Part model, mm, in its own coordinate system. Give positions to 0.01 mm unless a question says otherwise; leave off trailing zeros. Write each loop counter-clockwise with the first axis right and the second up, starting at its lowest first coordinate (ties: lowest second). Pieces come first, ordered by that corner, then holes. Notation, with made-up numbers: M 81.25,-31.5 L 96.25,-31.5 A30 cw 96.25,-3.5 Z; hole C 40,26 d10. An arc over 180 degrees is marked long. Use a Markdown table: item, result. Add a question column.
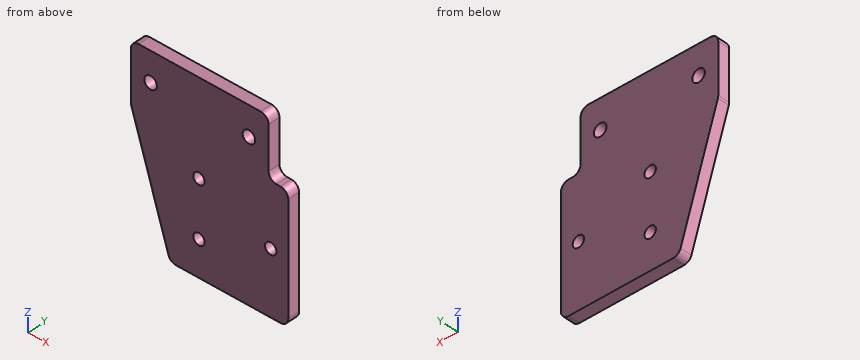
from build123d import *

# Parameters (mm, degrees)
SKETCH_1_R      = 1.6
SKETCH_1_R_2    = 1.45
EXTRUDE_1_DEPTH = 3
FILLET_2_R      = 2


with BuildPart() as part:
    # 草图1 → 凸台-拉伸1 (new body)
    with BuildSketch(Plane(origin=(0, 0, 0), x_dir=(1, 0, 0), z_dir=(0, 1, 0))):
        Polygon((0, 0), (0, 15), (10, 47), (25, 47), (40, 47), (40, 15), (35, 15), (35, 0), align=None)
        with Locations(Location((30, 7.5, 0), (0, 0, 270))):
            Circle(SKETCH_1_R, mode=Mode.SUBTRACT)
        with Locations(Location((5, 7.5, 0), (0, 0, 90))):
            Circle(SKETCH_1_R, mode=Mode.SUBTRACT)
        with Locations(Location((35.551575044, 30.824296308, 0), (0, 0, 270))):
            Circle(SKETCH_1_R_2, mode=Mode.SUBTRACT)
        with Locations(Location((17.301575044, 37.924296308, 0), (0, 0, 270))):
            Circle(SKETCH_1_R_2, mode=Mode.SUBTRACT)
        with Locations(Location((17.301575044, 23.724296308, 0), (0, 0, 270))):
            Circle(SKETCH_1_R_2, mode=Mode.SUBTRACT)
    extrude(amount=EXTRUDE_1_DEPTH)

    # 圆角2
    fillet_2_edges = [part.edges().sort_by_distance(p)[0] for p in [
        (35, 1.5, -15),
        (35, 1.5, 0),
        (0, 1.5, 0),
        (0, 1.5, -15),
        (10, 1.5, -47),
        (40, 1.5, -47),
        (40, 1.5, -15),
    ]]
    fillet(fillet_2_edges, radius=FILLET_2_R)


solid = part.part
1. Flat gauge pins, fed straight in: pin 1 (1 mm diameter, centred on y = 2.5, z = -23.5, fed in from -X); pin 2 (2.5 mm diameter, centred on x = 17.3, z = -37.92, fed in from -Y); pin 3 (1.1 mm diameter, centred on x = 37.5, y = 2, fed in from +Z); pin 4 (1.5 mm diameter, centred on y = 1.5, z = -23, fed in from -X). Where does each tip first touch, or does it go through?
2. Cut at C-C (y = 0.5). Write the cut outline in (x, z), then the cut area to 3 significant figures.
3. Drill centre lines: probe 1 along X at (y, z) = (2.2, -7.5); probe 2 along X at (y, z) = (2.25, -8); probe 3 along X at (y, z) = (0.4, -30). Where is each one in solid material? Low to high. Write a range as [from, to].
4. Cut at B-B (z = -7.5). Write the cut outline in (x, y).
5. Cut at A-A (x = 5). Write the cut outline in (y, z), then the cut area to 3 significant figures.
6. Cut at D-D (x = 30). Write the cut outline in (y, z).
A:
| question | item | result |
|---|---|---|
| 1 | pin 1 | stops at x = 2.5 |
| 1 | pin 2 | passes through |
| 1 | pin 3 | stops at z = -15 |
| 1 | pin 4 | stops at x = 2.27 |
| 2 | outline | M 0,-14.69 A2 ccw 0.09,-15.29 L 9.56,-45.6 A2 ccw 11.47,-47 L 38,-47 A2 ccw 40,-45 L 40,-17 A2 ccw 38,-15 L 37,-15 A2 cw 35,-13 L 35,-2 A2 ccw 33,0 L 2,0 A2 ccw 0,-2 Z; hole C 5,-7.5 d3.2; hole C 17.3,-37.92 d2.9; hole C 17.3,-23.72 d2.9; hole C 30,-7.5 d3.2; hole C 35.55,-30.82 d2.9 |
| 2 | area | 1,610 mm² |
| 3 | probe 1 | x = [0, 3.4], [6.6, 28.4], [31.6, 35] |
| 3 | probe 2 | x = [0, 3.48], [6.52, 28.48], [31.52, 35] |
| 3 | probe 3 | x = [4.69, 34.36], [36.74, 40] |
| 4 | outline | M 0,0 L 3.4,0 L 3.4,3 L 0,3 Z; M 6.6,0 L 28.4,0 L 28.4,3 L 6.6,3 Z; M 31.6,0 L 35,0 L 35,3 L 31.6,3 Z |
| 5 | outline | M 0,-31 L 3,-31 L 3,-9.1 L 0,-9.1 Z; M 0,-5.9 L 3,-5.9 L 3,0 L 0,0 Z |
| 5 | area | 83.4 mm² |
| 6 | outline | M 0,-47 L 3,-47 L 3,-9.1 L 0,-9.1 Z; M 0,-5.9 L 3,-5.9 L 3,0 L 0,0 Z |
